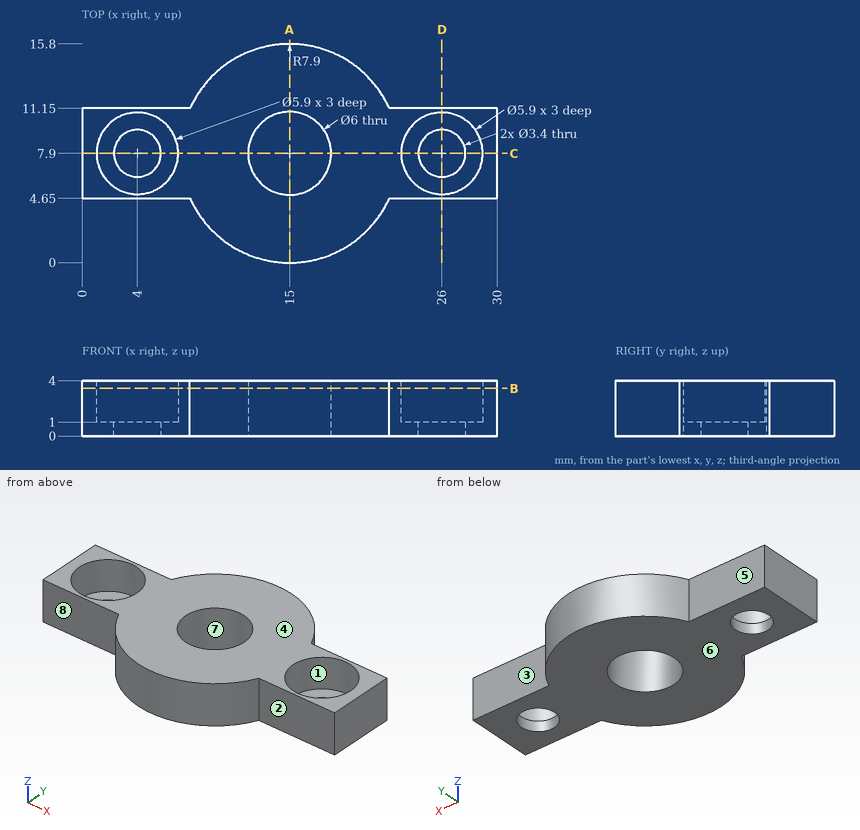
Answer from the drawing. Dimensions are ordinates in mm from the lowest x, y and z of the part. A direction names the side the tool comes from. Give positions to 0.01 mm unless a question says otherwise; leave off trailing zeros. Write each loop counter-clockwise with the first axis right and the second up, starting at its lowest first coordinate (ties: lowest second). Pieces come first, ordered by that corner, then holes. Notation, with made-up numbers: (83, 66.25) -> (118, 66.25) arc R10 cw to (118, 72.25) -> close; hole circle Ø11 at (63.5, 45.25). An arc over 180 degrees is marked (long way). Use a Markdown table: item, result.
(1) For the marked faces 1, 2, 3, 4 and 5, determine the directions among +Z, -Z, +X, -X, +Y, -Y from which every point of the face is accessible in a straight line to the end or side of a thin tool.
Return value:
| item | result |
|---|---|
| face 1 | +Z |
| face 2 | +Z, -Z, +X, -Y |
| face 3 | +Z, -Z, +X, +Y |
| face 4 | +Z, +X, -X, +Y, -Y |
| face 5 | +Z, -Z, -X, +Y |
(2) Section C-C, the plane y = 7.9 is taken. Determine the outline of the cut face in (x, z).
Return value:
| item | result |
|---|---|
| outline | (0, 0) -> (2.3, 0) -> (2.3, 1) -> (1.05, 1) -> (1.05, 4) -> (0, 4) -> close; (5.7, 0) -> (12, 0) -> (12, 4) -> (6.95, 4) -> (6.95, 1) -> (5.7, 1) -> close; (18, 0) -> (24.3, 0) -> (24.3, 1) -> (23.05, 1) -> (23.05, 4) -> (18, 4) -> close; (27.7, 0) -> (30, 0) -> (30, 4) -> (28.95, 4) -> (28.95, 1) -> (27.7, 1) -> close |
(3) Flat-ended cylindrical pins translate along their axes: P1, Ø8, axis at x = 15, y = 7.9, coming from the -Z side; P2, Ø5.5, axis at x = 26, y = 7.9, coming from the +Z side; P3, Ø2, axis at x = 21.5, z = 3, coming from the -Y side; P4, Ø2, axis at x = 28, z = 2.5, coming from the -Y side. Find the tip coordinate at first contact, or state that the pin passes through.
Return value:
| item | result |
|---|---|
| P1 | z = 0 |
| P2 | z = 1 |
| P3 | y = 2.23 |
| P4 | y = 4.65 |
(4) Determine the mould class of the marked faces 6, 7 and 8 for opening direction Y: released by +Y, released by -Y, zero draft, split by the parting line, or undercut.
Return value:
| item | result |
|---|---|
| face 6 | zero draft |
| face 7 | undercut |
| face 8 | released by -Y |
(5) Section D-D, the plane x = 26 is taken. Determine the outline of the cut face in (y, z).
Return value:
| item | result |
|---|---|
| outline | (4.65, 0) -> (6.2, 0) -> (6.2, 1) -> (4.95, 1) -> (4.95, 4) -> (4.65, 4) -> close; (9.6, 0) -> (11.15, 0) -> (11.15, 4) -> (10.85, 4) -> (10.85, 1) -> (9.6, 1) -> close |
(6) Find the intervals of material crossed by probe 1 along Y at (x, z) = (26, 3.25); probe 2 along X at (y, z) = (7.5, 3.05); probe 3 along Y at (x, z) = (15, 1.7), in increasing order. Write a range as from..to.
Return value:
| item | result |
|---|---|
| probe 1 | 4.65..4.95, 10.85..11.15 |
| probe 2 | 0..1.08, 6.92..12.03, 17.97..23.08, 28.92..30 |
| probe 3 | 0..4.9, 10.9..15.8 |
(7) Section A-A, the plane x = 15 is taken. Determine the outline of the cut face in (y, z), then the cut area to 3 significant figures.
Return value:
| item | result |
|---|---|
| outline | (0, 0) -> (4.9, 0) -> (4.9, 4) -> (0, 4) -> close; (10.9, 0) -> (15.8, 0) -> (15.8, 4) -> (10.9, 4) -> close |
| area | 39.2 mm2 |
(8) Section B-B, the plane z = 3.45 is taken. Determine the outline of the cut face in (x, y), then the cut area to 3 significant figures.
Return value:
| item | result |
|---|---|
| outline | (0, 4.65) -> (7.8, 4.65) arc R7.9 ccw to (22.2, 4.65) -> (30, 4.65) -> (30, 11.15) -> (22.2, 11.15) arc R7.9 ccw to (7.8, 11.15) -> (0, 11.15) -> close; hole circle Ø5.9 at (4, 7.9); hole circle Ø6 at (15, 7.9); hole circle Ø5.9 at (26, 7.9) |
| area | 208 mm2 |
